Could you check a few things on this model? Use its own coordinates, in mm. Face numbers are marked on the shaded views. Round coordinates to 2 decimals unless told otherwise and drop trailing zeros. Loops run counter-clockwise (first coordinate to the right, second up) from the corner with the lowest first, then second, coordinate; pieces in that order, holes last. Notation, with made-up numbers: (-33.75, 49) -> (-27.75, 49) arc R19 cw to (-27.75, 86) -> close; hole circle Ø2 at (-9.75, 14.25). An arc over 180 degrees is marked (long way). One line per item, written item: value.
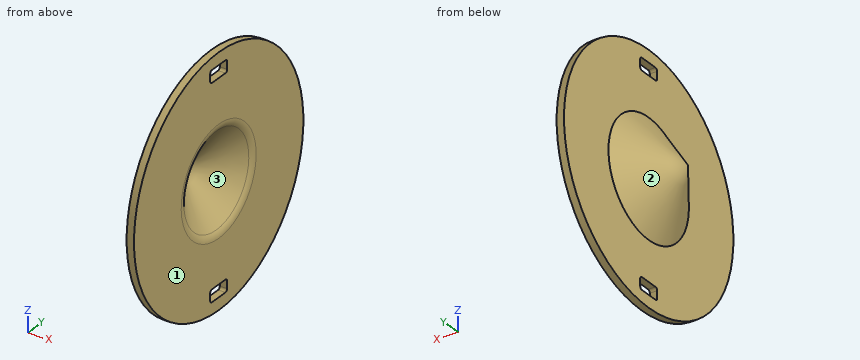
Autodesk Fusion 360 part; units mm, degrees
sketch "Sketch1" plane through (0, 0, 0) normal (0, 1, 0) x (1, 0, 0)
  line L0 (0, 0) -> (0, 23.75)
  line L1 (0, 0) -> (0, 50)
  line L2 (0, 50) -> (3, 50)
  line L3 (3, 50) -> (3, 0)
  line L4 (0, 0) -> (-16.0313, 0)
  line L5 (0, 23.75) -> (-16.0313, 0)
  line L6 (3, 0) -> (0, 0)
  dimension "d1" = 23.75
  dimension "d2" = 3
  dimension "d3" = 16.0313
revolve "Revolve1" add sketch "Sketch1" angle 360 about axis through (0, 0, 0) along (-1, 0, 0) contours L0 L1 L4 L5
revolve "Revolve2" add sketch "Sketch1" angle 360 about axis through (3, 0, 0) along (-1, 0, 0) contours L0 L1 L2 L3 L6
sketch "Sketch2" plane through (0, 0, 0) normal (0, 1, 0) x (1, 0, 0)
  line L0 (0, 0) -> (3, 0)
  line L1 (3, 0) -> (-12, 0)
  line L2 (3, 0) -> (3, 20.5)
  line L3 (3, 20.5) -> (-12, 0)
  line L4 (3, 20.5) -> (3, 0)
  dimension "d6" = 3
  dimension "d7" = 15
  dimension "d8" = 20.5
revolve "Revolve3" cut sketch "Sketch2" angle 360 about axis through (1.75, 0, 0) along (1, 0, 0)
sketch "Sketch3" plane through (3, 0, 0) normal (1, 0, 0) x (0, 0, -1)
  circle A0 centre (0, 0) radius 50
  line L0 (0, 0) -> (0, 5)
  line L1 (0, 5) -> (0, -5)
  line L2 (0, 5) -> (-45, 5)
  line L3 (0, -5) -> (-45, -5)
  line L4 (-45, 5) -> (-45, -5)
  line L5 (-45, 5) -> (-40, 5)
  line L6 (-40, 5) -> (-40, -5)
  line L7 (-40, -5) -> (-45, -5)
  line L8 (-45, -5) -> (-45, 5)
  line L9 (40, 5) -> (40, -5)
  line L10 (0, 5) -> (45, 5)
  line L11 (45, -5) -> (45, 5)
  line L12 (40, -5) -> (45, -5)
  line L13 (0, -5) -> (45, -5)
  circle A1 centre (0, 0) radius 20.5
  dimension "d16" = 5
  dimension "d17" = 10
  dimension "d18" = 45
  dimension "d19" = 5
extrude "Extrude2" cut sketch "Sketch3" against normal blind 3 contours L2 L3 L4 L5 L6 L7 L8 | L9 L10 L11 L12 L13
fillet "Fillet2" radius 1 8 edges at (1.5, 5, 45) (1.5, 5, 40) (1.5, -5, 40) (1.5, -5, 45) (1.5, 5, -45) (1.5, 5, -40) (1.5, -5, -40) (1.5, -5, -45)
fillet "Fillet3" radius 5 1 edges at (3, 7.4131, 19.1127)
equation "d1 = ( 47.5 / 2 ) * 1 mm"
equation "d3 = ( 1.60313 * 10 ) * 1 mm"
equation "d7 = 18.000 mm - 3 mm"
equation "d8 = 23.5 mm - 3 mm"
Item 1: I need wall thicknesses on line 1 (Z direction, x = 0.5, y = 2.5); line 2 (X direction, y = 45, z = 16); line 3 (Z direction, x = 1.5, y = -8). Which ranges of each line are inside material? Lowest first, please. Write a range as from..to.
Output:
line 1: z = -49.94..-45, -40..-16.9, 16.9..40, 45..49.94
line 2: x = 0..3
line 3: z = -49.36..-16.63, 16.63..49.36
Item 2: If we section it at B-B on y = 40: List the corners of the cut face in (x, z) for me.
Output:
outline: (0, -30) -> (3, -30) -> (3, 30) -> (0, 30) -> close
Item 3: If we mould it in two halves opening along Y, with no side actions, what happens to the marked faces 1, 2 and 3? For each: released by +Y, released by -Y, zero draft, split by the parting line, or undercut.
Output:
face 1: zero draft
face 2: split by the parting line
face 3: undercut
Item 4: If we section it at C-C on z = 26: List the corners of the cut face in (x, y) for me, plus the area to 3 significant figures.
Output:
outline: (0, -42.71) -> (3, -42.71) -> (3, 42.71) -> (0, 42.71) -> close
area: 256 mm²
Item 5: Will these pins go through, and if not, where does the flat tip stop? pin 1 Ø1 at (x, y) = (-1, 0.5) entering from +Z; pin 2 Ø8 at (x, z) = (0.5, -29.5) entering from +Y; pin 3 Ø1.5 at (x, y) = (1, 1.5) entering from -Z; pin 4 Ø3.5 at (x, y) = (1, -1) entering from +Z.
Output:
pin 1: stops at z = 23
pin 2: stops at y = 43.01
pin 3: stops at z = -49.99
pin 4: stops at z = 50
Item 6: If we section it at D-D on x = -8: List the corners of the cut face in (y, z) for me, plus the area to 3 significant figures.
Output:
outline: circle Ø23.8 at (0, 0); hole circle Ø10.93 at (0, 0)
area: 351 mm²
Item 7: If we section it at A-A on x = -2.75: List the corners of the cut face in (y, z) for me.
Output:
outline: circle Ø39.35 at (0, 0); hole circle Ø25.28 at (0, 0)
